```python
from build123d import *

# Parameters (mm, degrees)
SKETCH023_W                     = 50
SKETCH023_H                     = 50
PAD005_DEPTH                    = 10
SKETCH024_W                     = 42
SKETCH024_H                     = 42
POCKET014_DEPTH                 = 7
SKETCH025_R                     = 11
POCKET015_DEPTH                 = 3.001
SKETCH022_R                     = 2
POCKET016_DEPTH                 = 5
PAD006_DEPTH                    = 10
POCKET017_DEPTH                 = 216.156281
POCKET017_LINEARPATTERN_2_DEPTH = 216.156281
LINEARPATTERN001_COUNT          = 2
LINEARPATTERN001_PITCH          = 18
FILLET002_R                     = 5


with BuildPart() as part:
    # Sketch023 → Pad005 (new body)
    with BuildSketch(Plane.XY):
        Rectangle(SKETCH023_W, SKETCH023_H)
    extrude(amount=PAD005_DEPTH)

    # Sketch024 (on Face6 of Pad005) → Pocket014 (cut)
    with BuildSketch(Plane.XY.offset(10)):
        Rectangle(SKETCH024_W, SKETCH024_H)
    extrude(amount=-POCKET014_DEPTH, mode=Mode.SUBTRACT)

    # Sketch025 (on Face11 of Pocket014) → Pocket015 (cut, through all)
    with BuildSketch(Plane.XY.offset(3)):
        Circle(SKETCH025_R)
    extrude(amount=-POCKET015_DEPTH, mode=Mode.SUBTRACT)

    # Sketch022 → Pocket016 (cut)
    with BuildSketch(Plane.XY.offset(5)):
        with Locations((-15.5, 15.5)):
            Circle(SKETCH022_R)
        with Locations((15.5, 15.5)):
            Circle(SKETCH022_R)
        with Locations((15.5, -15.5)):
            Circle(SKETCH022_R)
        with Locations((-15.5, -15.5)):
            Circle(SKETCH022_R)
    extrude(amount=-POCKET016_DEPTH, mode=Mode.SUBTRACT)

    # Sketch026 → Pad006 (join)
    with BuildSketch(Plane.XY):
        Polygon((-25, 25), (25, 25), (25, -25), (35, -7.679492), (35, 50), (-35, 50), (-35, -7.679492), (-25, -25), align=None)
    extrude(amount=PAD006_DEPTH)

    # Sketch021 → Pocket017 (cut, through all)
    with BuildSketch(Plane.XY):
        with BuildLine():
            ThreePointArc((-30, 15), (-28, 13), (-26, 15))
            Line((-26, 15), (-26, 25))
            ThreePointArc((-26, 25), (-28, 27), (-30, 25))
            Line((-30, 15), (-30, 25))
        make_face()
    pocket017 = extrude(amount=POCKET017_DEPTH, mode=Mode.SUBTRACT)

    # Sketch021 LinearPattern 2 → Pocket017 LinearPattern 2 (cut, through all)
    with BuildSketch(Plane(origin=(56, 0, 0), x_dir=(1, 0, 0), z_dir=(0, 0, 1))):
        with BuildLine():
            ThreePointArc((-30, 15), (-28, 13), (-26, 15))
            Line((-26, 15), (-26, 25))
            ThreePointArc((-26, 25), (-28, 27), (-30, 25))
            Line((-30, 15), (-30, 25))
        make_face()
    pocket017_linearpattern_2 = extrude(amount=POCKET017_LINEARPATTERN_2_DEPTH, mode=Mode.SUBTRACT)

    # LinearPattern001: Pocket017, Pocket017 LinearPattern 2 ×2
    with Locations(*[(0, i * LINEARPATTERN001_PITCH, 0) for i in range(1, LINEARPATTERN001_COUNT)]):
        add(pocket017, mode=Mode.SUBTRACT)
        add(pocket017_linearpattern_2, mode=Mode.SUBTRACT)

    # Fillet002
    fillet002_edges = [part.edges().sort_by_distance(p)[0] for p in [
        (25, -25, 5),
        (35, -7.679492, 5),
        (35, 50, 5),
        (-25, -25, 5),
        (-35, -7.679492, 5),
        (-35, 50, 5),
    ]]
    fillet(fillet002_edges, radius=FILLET002_R)


with BuildPart() as part_1:
    # Body007 placement: moved
    add(part.part.moved(Location((0, 0, 232.808))))


solid = part_1.part
```
Could you check a few things on this model? Use its own coordinates, in mm. A direction names the side the tool comes from. Round coordinates to 2 decimals unless told otherwise and drop trailing zeros. Write each loop counter-clockwise with the first axis right and the second up, starting at its lowest first coordinate (ties: lowest second). Pieces come first, ordered by that corner, then holes.
(1) Suppose I cut it at B-B on x = -28. Write out the boundary of the cut face in (y, z).
Findings below:
outline: (-19.8, 232.81) - (13, 232.81) - (13, 242.81) - (-19.8, 242.81) - close; (27, 232.81) - (31, 232.81) - (31, 242.81) - (27, 242.81) - close; (45, 232.81) - (50, 232.81) - (50, 242.81) - (45, 242.81) - close
(2) Suppose I cut it at A-A on y = 37. Write out the boundary of the cut face in (x, z).
Findings below:
outline: (-35, 232.81) - (-30, 232.81) - (-30, 242.81) - (-35, 242.81) - close; (-26, 232.81) - (26, 232.81) - (26, 242.81) - (-26, 242.81) - close; (30, 232.81) - (35, 232.81) - (35, 242.81) - (30, 242.81) - close
(3) Thinking about a two-plate mould opening in Y: for faces 4 (the face through (35, 19, 238)), 5 (the face through (-30.442, -15.574, 237.738)), 6 (the face through (-26, 20, 238)), which applies, +Y half, -Y half, draft (parallel to the pull), parting line (faces both ways), or undercut?
Findings below:
face 4: draft
face 5: -Y half
face 6: undercut
(4) Suppose I cut it at C-C on y = 0. Write out the boundary of the cut face in (x, z), and give its area (3 significant figures).
Findings below:
outline: (-35, 232.81) - (-11, 232.81) - (-11, 235.81) - (-21, 235.81) - (-21, 242.81) - (-35, 242.81) - close; (11, 232.81) - (35, 232.81) - (35, 242.81) - (21, 242.81) - (21, 235.81) - (11, 235.81) - close
area: 340 mm2
(5) Which directions (+Z, -Z, +X, -X, +Y, -Y) give clear straight access to the entire face, cutting with the end or side of a thin tool? Please do faces 1 (the face through (0, -25, 238)), 2 (the face through (-30, 38, 238)), 3 (the face through (-21, 0, 239)).
Findings below:
face 1: +Z, -Z, +X, -X, -Y
face 2: +Z, -Z
face 3: +Z
(6) Suppose I cut it at D-D on z = 237.5. State how many separate pieces and enclosed holes the cut face has, and give its area (3 significant figures).
Findings below:
separate pieces: 1
enclosed holes: 5
area: 3,090 mm2
(7) If I drill on probe 1 along X at (y, z) = (37, 237.5); probe 2 along Y at (x, z) = (3, 239.5); probe 3 along Z at (x, y) = (18.5, 17), over which ranges is the centre line in solid material (lowest first)?
Findings below:
probe 1: x = -35 to -30, -26 to 26, 30 to 35
probe 2: y = -25 to -21, 21 to 50
probe 3: z = 232.81 to 235.81
(8) For pin 1 (21 mm diameter, centred on x = 8.5, y = -10, fed in from +Z); pin 2 (5 mm diameter, centred on y = -17, z = 239.5, fed in from +X), each with a flat end and sliding along its axis, tell me the tip position at first contact or that it passes through.
Findings below:
pin 1: stops at z = 235.81
pin 2: stops at x = 31.06
